```python
from build123d import *

# Parameters (mm, degrees)
SKETCH1_R              = 11
BODY_DEPTH             = 10
M4_CLEARANCE_HOLE1_D   = 4.5
ELEVATION_START        = 4
SKETCH10_W             = 50
SKETCH10_H             = 50
SKETCH10_R             = 2.25
SKETCH10_R_2           = 11
ELEVATION_DEPTH        = 4
SKETCH13_R             = 3.75
M4_SCREW_PLACE_DEPTH   = 4
SKETCH14_R             = 7.25
SPRING_HOLE_DEPTH      = 10
SKETCH15_W             = 11
SKETCH15_H             = 6
NUT_HOLE_DEPTH         = 20
SKETCH16_R             = 3.25
SHAFT_HOLE_DEPTH       = 13
SKETCH17_R             = 4
BRAKE_SCREW_HOLE_DEPTH = 20
SKETCH18_W             = 6
SKETCH18_H             = 11
BRAKE_NUT_HOLE_DEPTH   = 25
CHAMFER1_SIZE          = 1


with BuildPart() as part:
    # Sketch1 → Body (new, symmetric)
    with BuildSketch(Plane.XY):
        Polygon((25, -25), (-25, -25), (-45, -25), (-45, 20), (-25, 20), (-25, 25), (25, 25), (25, 20), (45, 20), (45, -25), align=None)
        Circle(SKETCH1_R, mode=Mode.SUBTRACT)
    extrude(amount=BODY_DEPTH, both=True)

    # M4 Clearance Hole1 (through all)
    with Locations(Plane(origin=(0, 0, -10), x_dir=(-1, 0, 0), z_dir=(0, 0, -1))):
        with Locations((0, 0), (-14.25, 14.25), (14.25, -14.25), (14.25, 14.25), (-14.25, -14.25)):
            Hole(M4_CLEARANCE_HOLE1_D / 2)

    # Sketch10 → Elevation (add)
    with BuildSketch(Plane.XY.offset(10).offset(ELEVATION_START)):
        Rectangle(SKETCH10_W, SKETCH10_H)
        with Locations(Location((-14.25, -14.25, 0), (0, 0, 180))):
            Circle(SKETCH10_R, mode=Mode.SUBTRACT)
        with Locations(Location((14.25, -14.25, 0), (0, 0, 180))):
            Circle(SKETCH10_R, mode=Mode.SUBTRACT)
        with Locations(Location((14.25, 14.25, 0), (0, 0, 180))):
            Circle(SKETCH10_R, mode=Mode.SUBTRACT)
        Circle(SKETCH10_R_2, mode=Mode.SUBTRACT)
        with Locations(Location((-14.25, 14.25, 0), (0, 0, 180))):
            Circle(SKETCH10_R, mode=Mode.SUBTRACT)
    extrude(amount=-ELEVATION_DEPTH)

    # Sketch13 → M4_Screw_Place (cut)
    with BuildSketch(Plane(origin=(0, 0, -10), x_dir=(-1, 0, 0), z_dir=(0, 0, -1))):
        with Locations((-14.25, 14.25)):
            Circle(SKETCH13_R)
        with Locations((14.25, 14.25)):
            Circle(SKETCH13_R)
        with Locations((14.25, -14.25)):
            Circle(SKETCH13_R)
        with Locations((-14.25, -14.25)):
            Circle(SKETCH13_R)
    extrude(amount=-M4_SCREW_PLACE_DEPTH, mode=Mode.SUBTRACT)

    # Sketch14 → Spring_Hole (cut)
    with BuildSketch(Plane(origin=(0, 20, 0), x_dir=(1, 0, 0), z_dir=(0, 1, 0))):
        with Locations(Location((-35, 0, 0), (0, 0, 180))):
            Circle(SKETCH14_R)
    spring_hole = extrude(amount=-SPRING_HOLE_DEPTH, mode=Mode.SUBTRACT)

    # Sketch15 → Nut_Hole (cut)
    with BuildSketch(Plane.ZY.offset(45)):
        Rectangle(SKETCH15_W, SKETCH15_H)
    nut_hole = extrude(amount=-NUT_HOLE_DEPTH, mode=Mode.SUBTRACT)

    # Sketch16 → Shaft_Hole (cut)
    with BuildSketch(Plane(origin=(0, 10, 0), x_dir=(1, 0, 0), z_dir=(0, 1, 0))):
        with Locations(Location((-35, 0, 0), (0, 0, 180))):
            Circle(SKETCH16_R)
    shaft_hole = extrude(amount=-SHAFT_HOLE_DEPTH, mode=Mode.SUBTRACT)

    # Sketch17 → Brake_Screw_Hole (cut)
    with BuildSketch(Plane.ZY.offset(45)):
        with Locations((0, -15)):
            Circle(SKETCH17_R)
    brake_screw_hole = extrude(amount=-BRAKE_SCREW_HOLE_DEPTH, mode=Mode.SUBTRACT)

    # Sketch18 → Brake_Nut_Hole (cut)
    with BuildSketch(Plane.XZ.offset(25)):
        with Locations((28, 0)):
            Rectangle(SKETCH18_W, SKETCH18_H)
    brake_nut_hole = extrude(amount=-BRAKE_NUT_HOLE_DEPTH, mode=Mode.SUBTRACT)

    # Mirror1: Spring_Hole, Nut_Hole, Shaft_Hole, Brake_Screw_Hole, Brake_Nut_Hole across plane
    add(spring_hole.mirror(Plane(origin=(0, 0, 0), x_dir=(0, 0, 1), z_dir=(1, 0, 0))), mode=Mode.SUBTRACT)
    add(nut_hole.mirror(Plane(origin=(0, 0, 0), x_dir=(0, 0, 1), z_dir=(1, 0, 0))), mode=Mode.SUBTRACT)
    add(shaft_hole.mirror(Plane(origin=(0, 0, 0), x_dir=(0, 0, 1), z_dir=(1, 0, 0))), mode=Mode.SUBTRACT)
    add(brake_screw_hole.mirror(Plane(origin=(0, 0, 0), x_dir=(0, 0, 1), z_dir=(1, 0, 0))), mode=Mode.SUBTRACT)
    add(brake_nut_hole.mirror(Plane(origin=(0, 0, 0), x_dir=(0, 0, 1), z_dir=(1, 0, 0))), mode=Mode.SUBTRACT)

    # Chamfer1
    chamfer1_edges = [part.edges().sort_by_distance(p)[0] for p in [
        (25, 22.5, -10),
        (35, 20, -10),
        (-27.75, 20, 0),
        (-35, 20, 10),
        (-35, 20, -10),
        (-25, 22.5, -10),
        (0, 25, -10),
        (27.75, 20, 0),
        (25, 25, 2),
        (25, 20, 0),
        (45, 20, 0),
        (-45, 20, 0),
        (-25, 20, 0),
        (-25, 25, 2),
        (35, 20, 10),
        (-25, -2.5, 10),
        (0, 25, 14),
        (25, -2.5, 10),
    ]]
    chamfer(chamfer1_edges, length=CHAMFER1_SIZE)


solid = part.part
```
Can you work these out from the model? Positions are in its coordinate system, mm. A direction names the side the tool comes from. Round coordinates to 2 decimals unless told otherwise and drop trailing zeros. Loops run counter-clockwise (first coordinate to the right, second up) from the corner with the lowest first, then second, coordinate; pieces in that order, holes last. Notation, with made-up numbers: M 23,37 L 28,37 A12 cw 28,49 Z; hole C -4.75,75.25 d6. An arc over 180 degrees is marked long. Answer as a JSON object with one key per item and string values. Group by question number.
Q1. Imagine slicing it at D-D, the plane x = -35. Please give me the cut outline in (y, z).
Q2. Imagine slicing it at C-C, the plane z = 0. Count the separate pieces of the cut face and the enclosed holes in it, then the cut area to 3 significant figures.
Q3. Imagine slicing it at B-B, the plane x = 14.25. Please give me the cut outline in (y, z), then the cut area to 3 significant figures.
Q4. On a 3-axis mill with a long thin cutter (end or side, diameter ignored), from which of +Z, -Z, +X, -X, +Y, -Y can I reach the whole of each face in a straight line? I mean faces 1 (the flat face through (-17, 14, -6)), 2 (the flat face through (-25, 5, 12)), 3 (the flat face through (-25, -11, 0)), 4 (the flat face through (-30, -8, -5.5)). Say none if no direction works.
Q5. Imagine slicing it at A-A, the plane y = 4. Please give me the cut outline in (x, z).
Q6. Will these pins go through, and if not, where does the flat tip stop? pin 1 (2 mm diameter, centred on x = -14.5, y = 15, fed in from -Z); pin 2 (12 mm diameter, centred on x = 39.5, z = 0.5, fed in from +Y); pin 3 (6 mm diameter, centred on x = 14.25, y = -14.25, fed in from -Z); pin 4 (8.5 mm diameter, centred on x = 35, z = 0, fed in from +Y).
Q7. Please list where these lines run through material, in increasing order: L1, parallel to X at y = -14.25, z = 3.25; L2, parallel to Y at x = 41, z = 0.
Q8. We'd pull the mould along Z, two halves only. Please class faces 5 (the flat face through (11.8, -14.2, -6)), 6 (the cylindrical face through (27.757, 14.563, 0.319)), 7 (the flat face through (25, 5, 12)): +Z half, -Z half, draft (parallel to the pull), parting line (faces both ways), or undercut.
Findings:
{
 "1": {"outline": "M -25,-10 L 19,-10 L 20,-9 L 20,-8.25 L 19,-7.25 L 10,-7.25 L 10,-3.25 L 3,-3.25 L 3,-5.5 L -3,-5.5 L -3,5.5 L 3,5.5 L 3,3.25 L 10,3.25 L 10,7.25 L 19,7.25 L 20,8.25 L 20,9 L 19,10 L -25,10 Z; hole C -15,0 d8"},
 "2": {"separate pieces": "7", "enclosed holes": "5", "area": "2,740 mm2"},
 "3": {"outline": "M -25,-10 L -18,-10 L -18,-6 L -16.5,-6 L -16.5,14 L -25,14 Z; M -12,-6 L -10.5,-6 L -10.5,-10 L 10.5,-10 L 10.5,-6 L 12,-6 L 12,14 L -12,14 Z; M 16.5,-6 L 18,-6 L 18,-10 L 24,-10 L 25,-9 L 25,13 L 24,14 L 16.5,14 Z", "area": "959 mm2"},
 "4": {"face 1": "-Z", "face 2": "+Z, -X, +Y", "face 3": "-Y", "face 4": "none"},
 "5": {"outline": "M -45,-10 L -10.25,-10 L -10.25,14 L -25,14 L -25,11 L -26,10 L -45,10 Z; M 10.25,-10 L 45,-10 L 45,10 L 26,10 L 25,11 L 25,14 L 10.25,14 Z; hole C -35,0 d6.5; hole C 35,0 d6.5"},
 "6": {"pin 1": "passes through", "pin 2": "stops at y = 20", "pin 3": "stops at z = -6", "pin 4": "stops at y = 10"},
 "7": {"L1": "x = -25 to -16.5, -12 to 12, 16.5 to 25", "L2": "y = -25 to -19, -11 to -3, 3 to 10"},
 "8": {"face 5": "-Z half", "face 6": "undercut", "face 7": "draft"}
}
